Check sheet for the drawn part. Datum: minimum x, y, z corner. Units: mm. A direction names the side the tool comes from. Give positions to 0.01 mm unless a question says otherwise; leave off trailing zeros. Write each loop counter-clockwise with the first axis right and the second up, starting at its lowest first coordinate (ties: lowest second). Pieces come first, ordered by that corner, then holes. Notation, with made-up numbers: M -17.5,45.5 L 12.5,45.5 A26 cw 12.5,82.5 Z; hole C 4.25,-22.5 d5. An arc over 180 degrees is marked long. Write item = value, one per line.
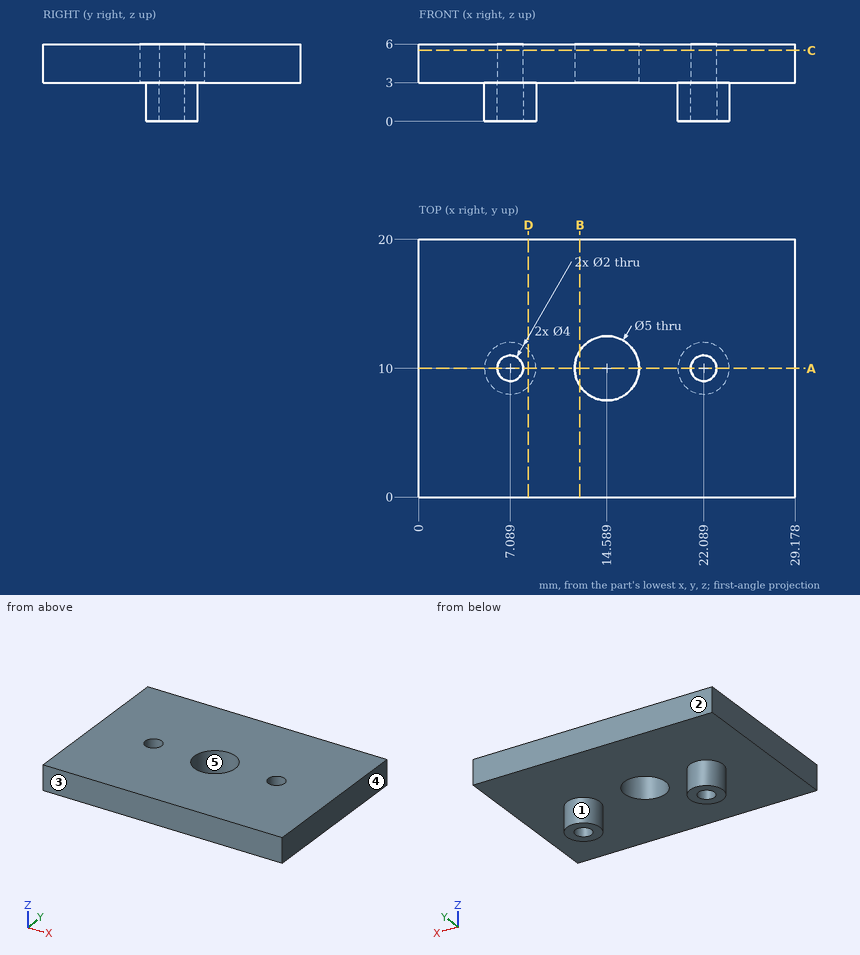
1) Cross-section at D-D on x = 8.5. Record the boundary of the cut face in (y, z), plus the area to 3 significant figures.
From the geometry:
outline = M 0,3 L 8.58,3 L 8.58,0 L 11.42,0 L 11.42,3 L 20,3 L 20,6 L 0,6 Z
area = 68.5 mm^2
2) Tool access check on the marked faces 1 and 2. Record the directions out of +Z, -Z, +X, -X, +Y, -Y that give a thin tool (end or side, any length) a straight path to the whole face; none if there is none.
From the geometry:
face_1 = -Z
face_2 = +Z, -Z, +X, -X, +Y
3) Cross-section at A-A on y = 10. Record the boundary of the cut face in (x, z).
From the geometry:
outline = M 0,3 L 5.09,3 L 5.09,0 L 6.09,0 L 6.09,6 L 0,6 Z; M 8.09,0 L 9.09,0 L 9.09,3 L 12.09,3 L 12.09,6 L 8.09,6 Z; M 17.09,3 L 20.09,3 L 20.09,0 L 21.09,0 L 21.09,6 L 17.09,6 Z; M 23.09,0 L 24.09,0 L 24.09,3 L 29.18,3 L 29.18,6 L 23.09,6 Z
4) Draft check along Y on the marked faces 3, 4 and 5. Enter one of: +Y half, -Y half, draft (parallel to the pull), parting line (faces both ways), or undercut.
From the geometry:
face_3 = -Y half
face_4 = draft
face_5 = undercut
5) Cross-section at B-B on x = 12.5. Record the boundary of the cut face in (y, z).
From the geometry:
outline = M 0,3 L 8.63,3 L 8.63,6 L 0,6 Z; M 11.37,3 L 20,3 L 20,6 L 11.37,6 Z
6) Material ranges on probe 1 along X at (y, z) = (10, 4.25); probe 2 along Y at (x, z) = (22, 1.3); probe 3 along Z at (x, y) = (23, 16.25), recorded low to high. Write a range as from..to.
From the geometry:
probe_1 = 0..6.09, 8.09..12.09, 17.09..21.09, 23.09..29.18
probe_2 = 8..9, 11..12
probe_3 = 3..6
7) Cross-section at C-C on z = 5.5. Record the boundary of the cut face in (x, y).
From the geometry:
outline = M 0,0 L 29.18,0 L 29.18,20 L 0,20 Z; hole C 7.09,10 d2; hole C 14.59,10 d5; hole C 22.09,10 d2
8) Depth check by flat-ended pin: P1, Ø6, axis at x = 16, y = 12.5, coming from the -Z side; P2, Ø1.8, axis at x = 7.09, y = 10, coming from the -Z side. Enter the tip coordinate at first touch or a pass-through.
From the geometry:
P1 = 3
P2 = through
